CAD build for the part. Positions are in the model's coordinates, mm. A direction names the side the tool comes from. Give positions to 0.01 mm unless a question says otherwise; leave off trailing zeros. Loops run counter-clockwise (first coordinate to the right, second up) from the corner with the lowest first, then second, coordinate; pieces in that order, holes last.
```python
from build123d import *

# Parameters (mm, degrees)
SKETCH2_R   = 9.525
SKETCH2_R_2 = 7.874


with BuildPart() as part:
    # Sweep1: sweep along a path in Sketch1
    with BuildLine(Plane.XY) as sweep1_path:
        Line((27.57027, 26.455034237), (68.338349684, 26.455034237))
        ThreePointArc((68.338349684, 26.455034237), (78.284445531, 25.803132673), (88.060360921, 23.8585822))
        Line((88.060360921, 23.8585822), (117.749211055, 15.903478782))
        ThreePointArc((117.749211055, 15.903478782), (127.525126444, 13.958928309), (137.471222292, 13.307026745))
        Line((137.471222292, 13.307026745), (193.607381659, 13.307026745))
        ThreePointArc((193.607381659, 13.307026745), (203.553477506, 13.958928309), (213.329392896, 15.903478782))
        Line((213.329392896, 15.903478782), (243.01824303, 23.8585822))
        ThreePointArc((243.01824303, 23.8585822), (252.79415842, 25.803132673), (262.740254267, 26.455034237))
        Line((262.740254267, 26.455034237), (356.976413635, 26.455034237))
        ThreePointArc((356.976413635, 26.455034237), (366.922509482, 27.1069358), (376.698424872, 29.051486273))
        Line((376.698424872, 29.051486273), (416.077365926, 39.603041728))
    # Sketch2 → Sweep1 (sweep)
    with BuildSketch(Plane(origin=(27.57027, 26.455034237, 0), x_dir=(0, 0, -1), z_dir=(1, 0, 0))):
        Circle(SKETCH2_R)
        Circle(SKETCH2_R_2, mode=Mode.SUBTRACT)
    sweep(path=sweep1_path.line)


solid = part.part
```
1. Saw through at A-A, the plane x = 291.5. List the corners of the cut face in (y, z) (3 decimals), and give its area (3 significant figures).
Responses:
outline: circle Ø19.05 at (26.455, 0); hole circle Ø15.748 at (26.455, 0)
area: 90.2 mm2
2. Probe line 1 along Y through (x, z) = (167.5, 0); line 2 along Z through (x, y) = (342.5, 26); line 3 along Y through (x, z) = (297, -0.5). List the from-to ranges inside material, lowest first.
Responses:
line 1: y = 3.78 to 5.43, 21.18 to 22.83
line 2: z = -9.51 to -7.86, 7.86 to 9.51
line 3: y = 16.94 to 18.6, 34.31 to 35.97
3. Pull direction X, two halves, no side cores. Call faces 4 (the face through (310.518, 33.094, -4.233)), 5 (the face through (394.219, 43.523, 1.24)), 6 (the face through (48.24, 35.9, 1.24)): released by +X, released by -X, zero draft, split by the parting line, or undercut.
Responses:
face 4: undercut
face 5: split by the parting line
face 6: zero draft
4. Drop flat-ended pins along their axis: pin 1 (10 mm diameter, centred on y = 37, z = -5, fed in from +X); pin 2 (2 mm diameter, centred on x = 128.5, z = 3, fed in from -Y); pin 3 (10 mm diameter, centred on y = 43.5, z = -0.5, fed in from +X). Give the stop position or say it passes through.
Responses:
pin 1: stops at x = 418.11
pin 2: stops at y = 4.44
pin 3: stops at x = 414.53
5. Tool access for faces 1 (the face through (27.57, 19, -4)), 2 (the face through (48.24, 34.26, 1.03)), 3 (the face through (165.93, 5.62, 1.71)): list every direction of +Z, -Z, +X, -X, +Y, -Y with a clear straight run to the whole face (end or side of a thin tool).
Responses:
face 1: +Z, -Z, -X, +Y, -Y
face 2: -X
face 3: none
